The model under review builds one solid part; all positions refer to its coordinate system, in mm. Face numbers are marked on the shaded views. A direction names the side the tool comes from. Give positions to 0.01 mm unless a question says otherwise; leave off trailing zeros. Order: outer loops, then holes, each group sorted by start corner. A loop starts at its lowest first (then second) coordinate and runs counter-clockwise, first axis right, second up. Notation, with made-up numbers: (-4, -10) -> (4, -10) arc R22 cw to (4, 24) -> close; hole circle Ø1 at (-27, 18). An arc over 180 degrees is marked (long way). Use one line per item in the form item = value.
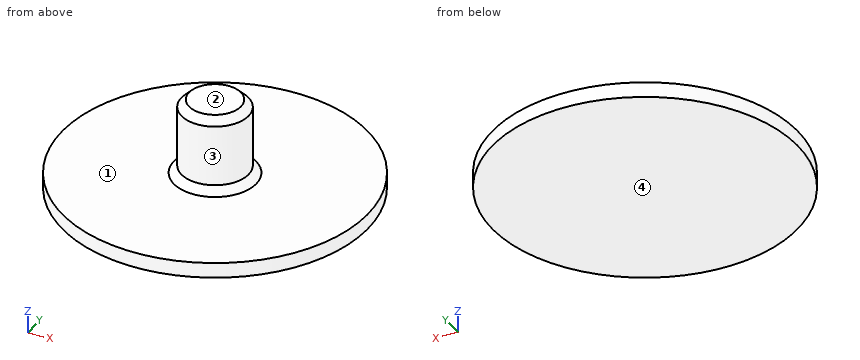
```python
from build123d import *

# Parameters (mm, degrees)
F0_R     = 10
F1_DEPTH = 1
F2_R     = 2.2
F3_DEPTH = 5
F4_SIZE  = 0.5


with BuildPart() as f1:
    # F0 (on Top) → F1 (new body)
    with BuildSketch(Plane.XY):
        Circle(F0_R)
    extrude(amount=F1_DEPTH)

    # F2 (on face) → F3 (join)
    with BuildSketch(Plane.XY.offset(1)):
        Circle(F2_R)
    extrude(amount=F3_DEPTH)

    # F4
    f4_edges = [f1.edges().sort_by_distance(p)[0] for p in [
        (-2.2, 0, 1),
        (-2.2, 0, 6),
    ]]
    chamfer(f4_edges, length=F4_SIZE)


solid = f1.part
```
1. For pin 1 Ø6 at (x, y) = (1, -5.5) entering from +Z; pin 2 Ø2 at (x, y) = (-3, -8) entering from -Z; pin 3 Ø1 at (x, z) = (0.5, 5) entering from +Y; pin 4 Ø1 at (x, y) = (7.5, 6.5) entering from +Z, all flat-tipped, find the tip position at first contact; note any pin that passes through.
Values:
pin_1 = 1.11
pin_2 = 0
pin_3 = 2.2
pin_4 = 1
2. For L1, parallel to Z at x = -8, y = -1.75; L2, parallel to X at y = 0.5, z = 2.35, list the stretches that pass through material, from the lowest coordinate up.
Values:
L1 = 0 to 1
L2 = -2.14 to 2.14
3. Add section D-D on x = 7.25. Give the boundary of the cut face in (y, z).
Values:
outline = (-6.89, 0) -> (6.89, 0) -> (6.89, 1) -> (-6.89, 1) -> close
4. The part is to be moulded in two halves that separate along X. For the marked faces 3 and 4, say which applies: +X half, -X half, draft (parallel to the pull), parting line (faces both ways), or undercut.
Values:
face_3 = parting line
face_4 = draft
5. Add section A-A on y = 0. Give the boundary of the cut face in (x, z).
Values:
outline = (-10, 0) -> (10, 0) -> (10, 1) -> (2.7, 1) -> (2.2, 1.5) -> (2.2, 5.5) -> (1.7, 6) -> (-1.7, 6) -> (-2.2, 5.5) -> (-2.2, 1.5) -> (-2.7, 1) -> (-10, 1) -> close
6. Add section C-C on z = 3. Give the boundary of the cut face in (x, y).
Values:
outline = circle Ø4.4 at (0, 0)
7. Tool access review of the marked faces 1 and 2: name each direction out of +Z, -Z, +X, -X, +Y, -Y from which nothing blocks a thin tool from reaching the whole face with its end or side.
Values:
face_1 = +Z
face_2 = +Z, +X, -X, +Y, -Y
